from build123d import *

# Parameters (mm, degrees)
CROQUIS1_R              = 2.5
SALIENTE_EXTRUIR1_DEPTH = 3
REDONDEO1_R             = 4
SALIENTE_EXTRUIR2_DEPTH = 15
CROQUIS3_W              = 9.109730849
CROQUIS3_H              = 7.453923598
SALIENTE_EXTRUIR3_DEPTH = 4
CROQUIS4_R              = 2.5
SALIENTE_EXTRUIR4_DEPTH = 13
CROQUIS5_W              = 20
CROQUIS5_H              = 4.5
CORTAR_EXTRUIR1_DEPTH   = 17
CORTAR_EXTRUIR2_DEPTH   = 6.5


with BuildPart() as part:
    # Croquis1 → Saliente-Extruir1 (new body)
    with BuildSketch(Plane(origin=(0, 0, 0), x_dir=(1, 0, 0), z_dir=(0, 1, 0))):
        with BuildLine():
            Line((-1.502919204, 4.425183821), (-1.502919204, -0.574816179))
            Line((-1.502919204, -0.574816179), (-3.752919204, -0.574816179))
            Line((-3.752919204, -0.574816179), (-3.752919204, -2.574816179))
            Line((-3.752919204, -2.574816179), (4.247080796, -2.574816179))
            Line((4.247080796, -2.574816179), (4.247080796, -0.574816179))
            Line((4.247080796, -0.574816179), (1.997080796, -0.574816179))
            Line((1.997080796, -0.574816179), (1.997080796, 4.425183821))
            Line((1.997080796, 4.425183821), (10.247080796, 4.425183821))
            Line((10.247080796, 4.425183821), (10.247080796, -9.382782341))
            Line((10.247080796, -9.382782341), (10.247080796, -20.574816179))
            Line((10.247080796, -20.574816179), (0.247080796, -20.574816179))
            ThreePointArc((0.247080796, -20.574816179), (-6.823987016, -17.645883991), (-9.752919204, -10.574816179))
            Line((-9.752919204, -10.574816179), (-9.752919204, 4.425183821))
            Line((-9.752919204, 4.425183821), (-1.502919204, 4.425183821))
        make_face()
        with Locations((0.247080796, -17.574816179)):
            Circle(CROQUIS1_R, mode=Mode.SUBTRACT)
    extrude(amount=SALIENTE_EXTRUIR1_DEPTH)

    # Redondeo1
    redondeo1_edges = [part.edges().sort_by_distance(p)[0] for p in [
        (10.247080796, 1.5, 20.574816179),
    ]]
    fillet(redondeo1_edges, radius=REDONDEO1_R)

    # Croquis2 → Saliente-Extruir2 (add)
    with BuildSketch(Plane(origin=(0, 3, 0), x_dir=(1, 0, 0), z_dir=(0, 1, 0))):
        Polygon((-9.752919204, -3.574816179), (10.247080796, -3.574816179), (10.247080796, 4.425183821), (1.997080796, 4.425183821), (1.997080796, -0.574816179), (4.247080796, -0.574816179), (4.247080796, -2.574816179), (-3.752919204, -2.574816179), (-3.752919204, -0.574816179), (-1.502919204, -0.574816179), (-1.502919204, 4.425183821), (-9.752919204, 4.425183821), align=None)
    extrude(amount=SALIENTE_EXTRUIR2_DEPTH)

    # Croquis3 → Saliente-Extruir3 (add)
    with BuildSketch(Plane.XZ):
        with Locations((0.202425252, -0.698222022)):
            Rectangle(CROQUIS3_W, CROQUIS3_H)
    extrude(amount=-SALIENTE_EXTRUIR3_DEPTH)

    # Croquis4 → Saliente-Extruir4 (add)
    with BuildSketch(Plane.XZ):
        with BuildLine():
            Line((-9.752919204, -4.425183821), (10.247080796, -4.425183821))
            Line((10.247080796, -4.425183821), (10.247080796, 16.574816179))
            ThreePointArc((10.247080796, 16.574816179), (9.075507921, 19.403243304), (6.247080796, 20.574816179))
            Line((6.247080796, 20.574816179), (0.247080796, 20.574816179))
            ThreePointArc((0.247080796, 20.574816179), (-6.823987016, 17.645883991), (-9.752919204, 10.574816179))
            Line((-9.752919204, 10.574816179), (-9.752919204, -4.425183821))
        make_face()
        with Locations((0.247080796, 17.574816179)):
            Circle(CROQUIS4_R, mode=Mode.SUBTRACT)
    extrude(amount=-SALIENTE_EXTRUIR4_DEPTH)

    # Croquis5 → Cortar-Extruir1 (cut)
    with BuildSketch(Plane.XY.offset(20.574816179)):
        with Locations((0.247080796, 6.75)):
            Rectangle(CROQUIS5_W, CROQUIS5_H)
    extrude(amount=-CORTAR_EXTRUIR1_DEPTH, mode=Mode.SUBTRACT)

    # Croquis6 → Cortar-Extruir2 (cut)
    with BuildSketch(Plane(origin=(0, 13, 0), x_dir=(1, 0, 0), z_dir=(0, 1, 0))):
        Polygon((-1.502919204, 4.425183821), (-1.502919204, -0.574816179), (-3.752919204, -0.574816179), (-3.752919204, -2.574816179), (4.247080796, -2.574816179), (4.247080796, -0.574816179), (1.997080796, -0.574816179), (1.997080796, 4.425183821), align=None)
    extrude(amount=-CORTAR_EXTRUIR2_DEPTH, mode=Mode.SUBTRACT)


solid = part.part
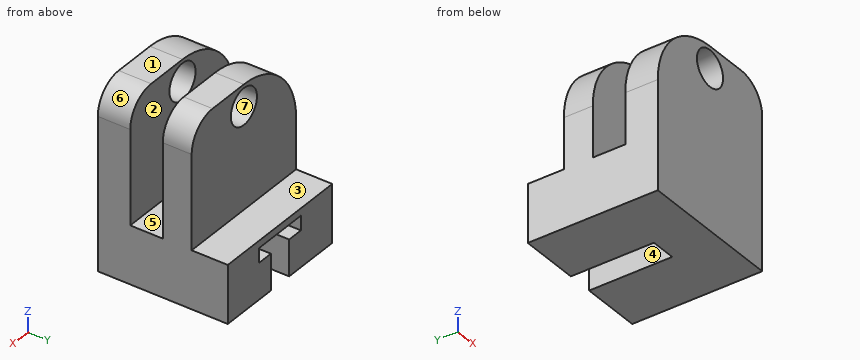
Source: CAD feature listing. Evaluate the final solid. Frame: model axes, mm. Face numbers are marked on the shaded views. A direction names the side the tool comes from. Round coordinates to 2 decimals unless told otherwise and drop trailing zeros. Loops run counter-clockwise (first coordinate to the right, second up) from the corner with the lowest first, then second, coordinate; pieces in that order, holes last.
Q1. Section B-B, the plane y = 14.5. Return loops of the section in (x, z).
Q2. Section A-A, the plane z = 8.5. Return loops of the section in (x, y).
Q3. Section C-C, the plane y = 11.75. Return loops of the section in (x, z), plus the area to 3 significant figures.
Q4. Ray query, line 1 (Y direction, x = -2.5, z = 10); line 2 (Z direction, x = -3.5, y = 13.5); line 3 (X direction, y = 16, z = -2.75). Return the intervals inside material, ascending.
Q5. Mould query, pull axis X, two halves, no side actions, for the marked faces 4, 5, 6 and 7. Classes: pulls with the +X half, pulls with the -X half, needs draft (parallel to the pull), parting line crosses it, or undercut.
Q6. Section D-D, the plane z = 18.25. Return loops of the section in (x, y).
Q7. First-contact query: P1, Ø4.5, axis at x = 0.25, z = 17.57, coming from the -Y side; P2, Ø1.5, axis at y = 13.5, z = 15.5, coming from the -X side; P3, Ø5, axis at x = -4.5, z = 13, coming from the +Y side; P4, Ø5.5, axis at x = -1, y = 16.5, coming from the +Z side. Flat tips, straight axial feed; report the tip coordinate or a pass-through.
Q8. Access query for the marked faces 1, 2 and 3. Directions: +Z, -Z, +X, -X, +Y, -Y. A direction counts if a zero-diameter tool reaches every point of the face in a straight line with its end or side. Return the directions, or none.
Solutions:
1. outline: (-9.75, -4.43) - (-1.5, -4.43) - (-1.5, 0.57) - (-3.75, 0.57) - (-3.75, 2.57) - (4.25, 2.57) - (4.25, 0.57) - (2, 0.57) - (2, -4.43) - (10.25, -4.43) - (10.25, 3.57) - (-9.75, 3.57) - close
2. outline: (-9.75, 0) - (10.25, 0) - (10.25, 4.5) - (-9.75, 4.5) - close; (-9.75, 9) - (10.25, 9) - (10.25, 13) - (-9.75, 13) - close
3. outline: (-9.75, -4.43) - (-1.5, -4.43) - (-1.5, 0.57) - (-3.75, 0.57) - (-3.75, 2.57) - (4.25, 2.57) - (4.25, 0.57) - (2, 0.57) - (2, -4.43) - (10.25, -4.43) - (10.25, 16.57) arc R4 ccw to (6.25, 20.57) - (0.25, 20.57) arc R10 ccw to (-9.75, 10.57) - close; hole circle Ø5 at (0.25, 17.57)
3. area: 422 mm2
4. line 1: y = 0 to 4.5, 9 to 13
4. line 2: z = -4.43 to 0.57, 2.57 to 3.57
4. line 3: x = -9.75 to -1.5, 2 to 10.25
5. face 4: undercut
5. face 5: needs draft
5. face 6: pulls with the +X half
5. face 7: undercut
6. outline: (-6.16, 0) - (-2.16, 0) - (-2.16, 4.5) - (-6.16, 4.5) - close; (-6.16, 9) - (-2.16, 9) - (-2.16, 13) - (-6.16, 13) - close; (2.65, 0) - (9.88, 0) - (9.88, 4.5) - (2.65, 4.5) - close; (2.65, 9) - (9.88, 9) - (9.88, 13) - (2.65, 13) - close
7. P1: passes through
7. P2: stops at x = -8.75
7. P3: stops at y = 13
7. P4: stops at z = 3.57
8. face 1: +Z, +X, -X, +Y, -Y
8. face 2: +Z, +X, -X
8. face 3: +Z, +X, -X, +Y
